from build123d import *

# Parameters (mm, degrees)
BOSS_EXTRUDE1_DEPTH = 10


with BuildPart() as part:
    # Sketch1 → Boss-Extrude1 (new body)
    with BuildSketch(Plane(origin=(0, 0, 0), x_dir=(0, 0, -1), z_dir=(1, 0, 0))):
        with BuildLine():
            ThreePointArc((22.695346806, 15.624541707), (15.572847807, 18.124541707), (22.695346806, 20.624541707))
            Line((22.695346806, 20.624541707), (25.027203864, 20.624541707))
            ThreePointArc((25.027203864, 20.624541707), (13.572847807, 18.124541707), (25.027203864, 15.624541707))
            Line((25.027203864, 15.624541707), (22.695346806, 15.624541707))
        make_face()
        with BuildLine():
            Line((25.027203864, 20.624541707), (22.695346806, 20.624541707))
            ThreePointArc((22.695346806, 20.624541707), (23.347102435, 19.449306592), (23.572847807, 18.124541707))
            ThreePointArc((23.572847807, 18.124541707), (23.347102435, 16.799776821), (22.695346806, 15.624541707))
            Line((22.695346806, 15.624541707), (25.027203864, 15.624541707))
            ThreePointArc((25.027203864, 15.624541707), (25.434849869, 16.84511534), (25.572847807, 18.124541707))
            ThreePointArc((25.572847807, 18.124541707), (25.434849869, 19.403968074), (25.027203864, 20.624541707))
        make_face()
        with BuildLine():
            Line((140.072847807, 20.624541707), (25.027203864, 20.624541707))
            ThreePointArc((25.027203864, 20.624541707), (25.434849869, 19.403968074), (25.572847807, 18.124541707))
            ThreePointArc((25.572847807, 18.124541707), (25.434849869, 16.84511534), (25.027203864, 15.624541707))
            Line((25.027203864, 15.624541707), (140.072847807, 15.624541707))
            Line((140.072847807, 15.624541707), (140.072847807, 20.624541707))
        make_face()
        with BuildLine():
            ThreePointArc((140.072847807, 20.624541707), (142.572847807, 18.124541707), (140.072847807, 15.624541707))
            Line((140.072847807, 15.624541707), (140.072847807, 20.624541707))
        make_face()
    extrude(amount=BOSS_EXTRUDE1_DEPTH)


solid = part.part
Geometry: final body of the model. Coordinates: model frame, mm. A direction names the side the tool comes from. Round coordinates to 2 decimals unless told otherwise and drop trailing zeros. Loops run counter-clockwise (first coordinate to the right, second up) from the corner with the lowest first, then second, coordinate; pieces in that order, holes last. Notation, with made-up numbers: (24.5, 48.5) -> (46.5, 48.5) arc R14 ccw to (46.5, 52.5) -> close; hole circle Ø11 at (43.25, -33.75). An arc over 180 degrees is marked (long way). One line per question, with ' | ' between items. Start each with the question number.
1. Section A-A on x = 5. Output: boundary loops of the cut face in (y, z).
2. Line query: line 1 along Y through (x, z) = (1.25, -128.5); line 2 along Z through (x, y) = (4.5, 19.5); line 3 along Z through (x, y) = (4, 20). Output: solid intervals per line, ascending. Write a range as [from, to].
3. Section B-B on z = -64. Output: boundary loops of the cut face in (x, y), and give its area (3 significant figures).
4. Set-up query: faces 1 (the face through (5, 15.625, -82)), 2 (the face through (4.93, 18.18, -142.572)), 3 (the face through (5, 20.625, -83)). Return all of +Z, -Z, +X, -X, +Y, -Y with unobstructed straight access to the full face (end or side cutting, diameter ignored); none if empty.
5. Contact query for flat-ended pins moving along their axis: pin 1 (2 mm diameter, centred on x = 3.5, y = 14, fed in from +Z); pin 2 (5 mm diameter, centred on x = 2.5, z = -58.5, fed in from +Y); pin 3 (3 mm diameter, centred on y = 15, z = -121, fed in from -X); pin 4 (2 mm diameter, centred on x = 5.5, y = 17, fed in from -Z). Output: stop coordinate, or through.
Returned:
1) outline: (15.62, -140.07) arc R2.5 ccw to (20.62, -140.07) -> (20.62, -25.03) arc R6 ccw (long way) to (15.62, -25.03) -> close; hole circle Ø8 at (18.12, -19.57)
2) line 1: y = [15.62, 20.62] | line 2: z = [-142.16, -23.33], [-15.82, -13.73] | line 3: z = [-141.73, -23.11], [-16.04, -13.87]
3) outline: (0, 15.62) -> (10, 15.62) -> (10, 20.62) -> (0, 20.62) -> close | area: 50.0 mm2
4) face 1: -Z, +X, -X, -Y | face 2: -Z, +X, -X | face 3: -Z, +X, -X, +Y
5) pin 1: stops at z = -14.45 | pin 2: stops at y = 20.62 | pin 3: stops at x = 0 | pin 4: stops at z = -142.57
